Source: three-view drawing plus pictorial views. Frame: mm from the lowest corner of the part. A direction names the side the tool comes from. Give positions to 0.01 mm unless a question says otherwise; leave off trailing zeros. Order: outer loops, then holes, each group sorted by start corner. A loop starts at its lowest first (then second) coordinate and runs counter-clockwise, first axis right, second up. Notation, with made-up numbers: (-1, -35.75) -> (29, -35.75) arc R11 ccw to (29, -14.75) -> close; hole circle Ø6 at (37, -21.5). An arc over 180 degrees is marked (long way). Answer in a Markdown table with one row per item.
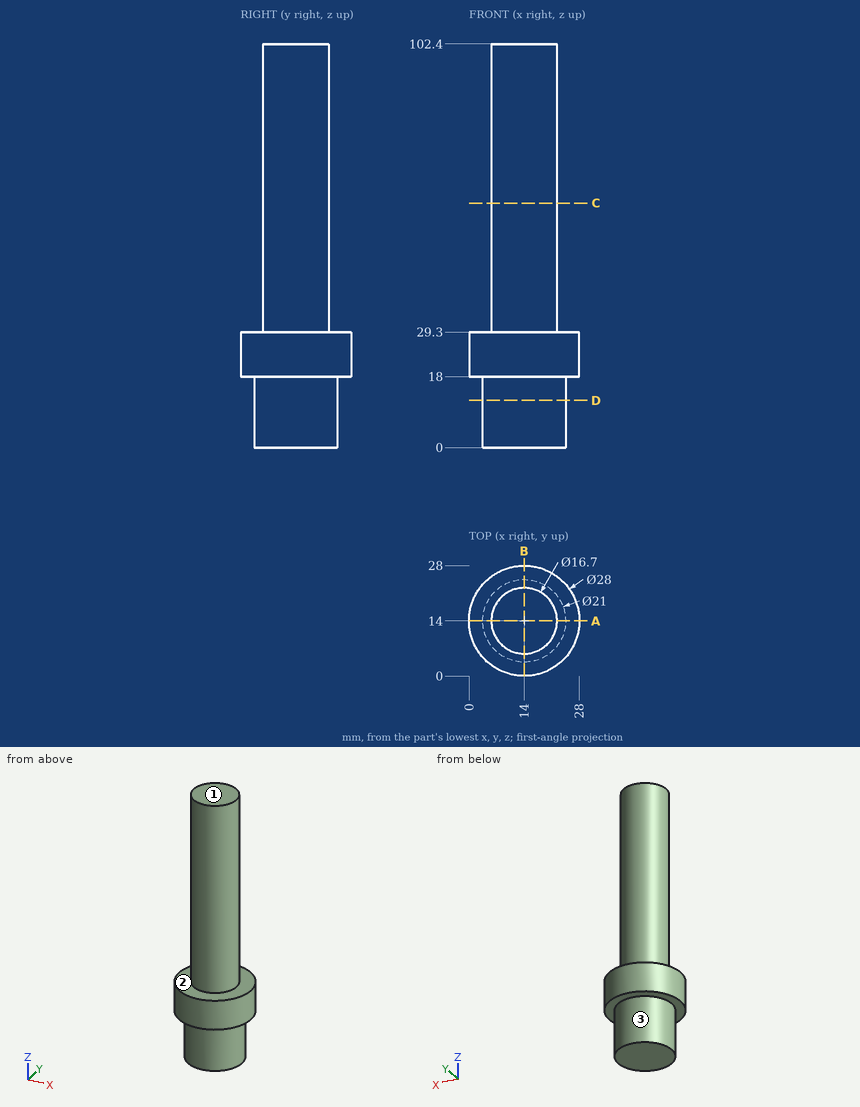
(1) Section query C-C (z = 62). Return the cut outline in (x, y).
A:
| item | result |
|---|---|
| outline | circle Ø16.7 at (14, 14) |
(2) Section query D-D (z = 12). Return the cut outline in (x, y), plus the area to 3 significant figures.
A:
| item | result |
|---|---|
| outline | circle Ø21 at (14, 14) |
| area | 346 mm^2 |
(3) Section query A-A (y = 14). Return the cut outline in (x, z).
A:
| item | result |
|---|---|
| outline | (0, 18) -> (3.5, 18) -> (3.5, 0) -> (24.5, 0) -> (24.5, 18) -> (28, 18) -> (28, 29.3) -> (22.35, 29.3) -> (22.35, 102.4) -> (5.65, 102.4) -> (5.65, 29.3) -> (0, 29.3) -> close |
(4) Ray query, probe 1 along X at (y, z) = (13.5, 9); probe 2 along Z at (x, y) = (3.25, 5.25); probe 3 along Z at (x, y) = (8.75, 6). Return the intervals inside material, ascending.
A:
| item | result |
|---|---|
| probe 1 | x = 3.51 to 24.49 |
| probe 2 | z = 18 to 29.3 |
| probe 3 | z = 0 to 29.3 |
(5) Access query for the marked faces 1, 2 and 3. Directions: +Z, -Z, +X, -X, +Y, -Y. A direction counts if a zero-diameter tool reaches every point of the face in a straight line with its end or side. Return the directions, or none.
A:
| item | result |
|---|---|
| face 1 | +Z, +X, -X, +Y, -Y |
| face 2 | +Z |
| face 3 | -Z |
(6) First-contact query: pin 1 Ø10 at (y, z) = (10.5, 38) entering from +X; pin 2 Ø1.5 at (y, z) = (21.5, 45) entering from +X; pin 3 Ø5 at (x, z) = (9.5, 76.5) entering from +Y. Flat tips, straight axial feed; report the tip coordinate or a pass-through.
A:
| item | result |
|---|---|
| pin 1 | stops at x = 22.35 |
| pin 2 | stops at x = 18.92 |
| pin 3 | stops at y = 22.11 |
